Verification items for the finished model (mm, model axes). Face numbers are marked on the shaded views. A direction names the side the tool comes from. Give positions to 0.01 mm unless a question says otherwise; leave off trailing zeros. Loops run counter-clockwise (first coordinate to the right, second up) from the corner with the lowest first, then second, coordinate; pieces in that order, holes last. Notation, with made-up numbers: M 28,-37 L 36,-37 A23 cw 36,-10 Z; hole C -14.5,-8 d5. An arc over 180 degrees is marked long. Use CSV: the item, a comma, the result in double quotes.
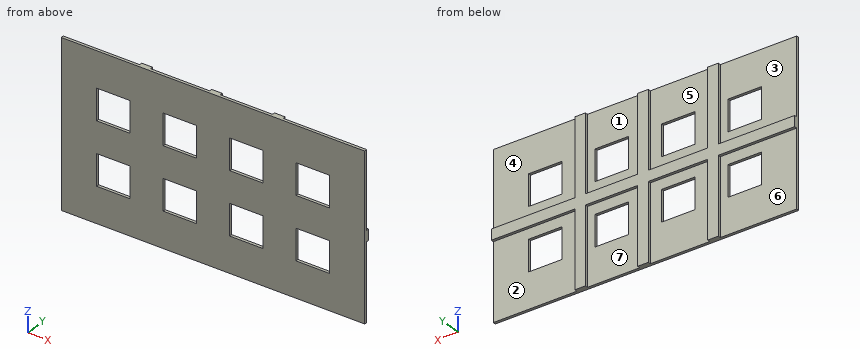
Autodesk Inventor part; units mm, degrees
ref_plane "YZ Plane" through (0, 0, 0) normal (1, 0, 0) x (0, 1, 0)
ref_plane "XZ Plane" through (0, 0, 0) normal (0, 1, 0) x (-1, 0, 0)
ref_plane "XY Plane" through (0, 0, 0) normal (0, 0, 1) x (1, 0, 0)
sketch "Sketch1" plane through (0, 0, 0) normal (0, 1, 0) x (-1, 0, 0)
  line L0 (0, 0) -> (-25.4, 0) construction
  line L1 (-25.4, 0) -> (-25.4, -25.4) construction
  line L2 (-25.4, -25.4) -> (0, -25.4) construction
  line L3 (0, -25.4) -> (0, 0) construction
  line L4 (-25.4, -25.4) -> (-49.2125, -25.4) construction
  line L5 (-49.2125, -25.4) -> (-49.2125, -47.625) construction
  line L6 (-49.2125, -47.625) -> (-25.4, -47.625) construction
  line L7 (-25.4, -47.625) -> (-25.4, -25.4) construction
  line L8 (-73.025, -25.4) -> (-96.8375, -25.4) construction
  line L9 (-96.8375, -25.4) -> (-96.8375, -47.625) construction
  line L10 (-96.8375, -47.625) -> (-73.025, -47.625) construction
  line L11 (-73.025, -47.625) -> (-73.025, -25.4) construction
  line L12 (-120.65, -25.4) -> (-144.4625, -25.4) construction
  line L13 (-144.4625, -25.4) -> (-144.4625, -47.625) construction
  line L14 (-144.4625, -47.625) -> (-120.65, -47.625) construction
  line L15 (-120.65, -47.625) -> (-120.65, -25.4) construction
  line L16 (-168.275, -25.4) -> (-192.0875, -25.4) construction
  line L17 (-192.0875, -25.4) -> (-192.0875, -47.625) construction
  line L18 (-192.0875, -47.625) -> (-168.275, -47.625) construction
  line L19 (-168.275, -47.625) -> (-168.275, -25.4) construction
  line L20 (-25.4, -69.85) -> (-49.2125, -69.85) construction
  line L21 (-49.2125, -69.85) -> (-49.2125, -92.075) construction
  line L22 (-49.2125, -92.075) -> (-25.4, -92.075) construction
  line L23 (-25.4, -92.075) -> (-25.4, -69.85) construction
  line L24 (-73.025, -69.85) -> (-96.8375, -69.85) construction
  line L25 (-96.8375, -69.85) -> (-96.8375, -92.075) construction
  line L26 (-96.8375, -92.075) -> (-73.025, -92.075) construction
  line L27 (-73.025, -92.075) -> (-73.025, -69.85) construction
  line L28 (-120.65, -69.85) -> (-144.4625, -69.85) construction
  line L29 (-144.4625, -69.85) -> (-144.4625, -92.075) construction
  line L30 (-144.4625, -92.075) -> (-120.65, -92.075) construction
  line L31 (-120.65, -92.075) -> (-120.65, -69.85) construction
  line L32 (-168.275, -69.85) -> (-192.0875, -69.85) construction
  line L33 (-192.0875, -69.85) -> (-192.0875, -92.075) construction
  line L34 (-192.0875, -92.075) -> (-168.275, -92.075) construction
  line L35 (-168.275, -92.075) -> (-168.275, -69.85) construction
  line L36 (-192.0875, -92.075) -> (-217.4875, -92.075) construction
  line L37 (-217.4875, -92.075) -> (-217.4875, -117.475) construction
  line L38 (-217.4875, -117.475) -> (-192.0875, -117.475) construction
  line L39 (-192.0875, -117.475) -> (-192.0875, -92.075) construction
  line L40 (0, 0) -> (-217.4875, 0)
  line L41 (-217.4875, 0) -> (-217.4875, -117.475)
  line L42 (-217.4875, -117.475) -> (0, -117.475)
  line L43 (0, -117.475) -> (0, 0)
  line L44 (-192.0875, -92.075) -> (-168.275, -92.075)
  line L45 (-168.275, -92.075) -> (-168.275, -69.85)
  line L46 (-168.275, -69.85) -> (-192.0875, -69.85)
  line L47 (-192.0875, -69.85) -> (-192.0875, -92.075)
  line L48 (-144.4625, -92.075) -> (-120.65, -92.075)
  line L49 (-120.65, -92.075) -> (-120.65, -69.85)
  line L50 (-120.65, -69.85) -> (-144.4625, -69.85)
  line L51 (-144.4625, -69.85) -> (-144.4625, -92.075)
  line L52 (-96.8375, -92.075) -> (-73.025, -92.075)
  line L53 (-73.025, -92.075) -> (-73.025, -69.85)
  line L54 (-73.025, -69.85) -> (-96.8375, -69.85)
  line L55 (-96.8375, -69.85) -> (-96.8375, -92.075)
  line L56 (-49.2125, -92.075) -> (-25.4, -92.075)
  line L57 (-25.4, -92.075) -> (-25.4, -69.85)
  line L58 (-25.4, -69.85) -> (-49.2125, -69.85)
  line L59 (-49.2125, -69.85) -> (-49.2125, -92.075)
  line L60 (-25.4, -47.625) -> (-49.2125, -47.625)
  line L61 (-49.2125, -47.625) -> (-49.2125, -25.4)
  line L62 (-49.2125, -25.4) -> (-25.4, -25.4)
  line L63 (-25.4, -25.4) -> (-25.4, -47.625)
  line L64 (-73.025, -47.625) -> (-96.8375, -47.625)
  line L65 (-96.8375, -47.625) -> (-96.8375, -25.4)
  line L66 (-96.8375, -25.4) -> (-73.025, -25.4)
  line L67 (-73.025, -25.4) -> (-73.025, -47.625)
  line L68 (-120.65, -47.625) -> (-144.4625, -47.625)
  line L69 (-144.4625, -47.625) -> (-144.4625, -25.4)
  line L70 (-144.4625, -25.4) -> (-120.65, -25.4)
  line L71 (-120.65, -25.4) -> (-120.65, -47.625)
  line L72 (-168.275, -47.625) -> (-192.0875, -47.625)
  line L73 (-192.0875, -47.625) -> (-192.0875, -25.4)
  line L74 (-192.0875, -25.4) -> (-168.275, -25.4)
  line L75 (-168.275, -25.4) -> (-168.275, -47.625)
  dimension "d1" = 25.4
  dimension "d2" = 23.8125
  dimension "d3" = 22.225
  dimension "d6" = 47.625
  dimension "d9" = 44.45
  dimension "d12" = 25.4
  dimension "d13" = 25.4
extrude "Extrusion1" add sketch "Sketch1" along normal blind 2
sketch "Sketch2" plane through (0, 2, 0) normal (0, 1, 0) x (1, 0, 0)
  line L0 (217.4875, 0) -> (217.4875, 117.475) construction
  line L1 (217.4875, 117.475) -> (0, 117.475) construction
  line L2 (0, 117.475) -> (0, 0) construction
  line L3 (0, 0) -> (217.4875, 0) construction
  line L4 (168.275, 47.625) -> (192.0875, 47.625) construction
  line L5 (192.0875, 47.625) -> (192.0875, 25.4) construction
  line L6 (192.0875, 25.4) -> (168.275, 25.4) construction
  line L7 (168.275, 25.4) -> (168.275, 47.625) construction
  line L8 (120.65, 47.625) -> (144.4625, 47.625) construction
  line L9 (144.4625, 47.625) -> (144.4625, 25.4) construction
  line L10 (144.4625, 25.4) -> (120.65, 25.4) construction
  line L11 (120.65, 25.4) -> (120.65, 47.625) construction
  line L12 (73.025, 47.625) -> (96.8375, 47.625) construction
  line L13 (96.8375, 47.625) -> (96.8375, 25.4) construction
  line L14 (96.8375, 25.4) -> (73.025, 25.4) construction
  line L15 (73.025, 25.4) -> (73.025, 47.625) construction
  line L16 (25.4, 47.625) -> (49.2125, 47.625) construction
  line L17 (49.2125, 47.625) -> (49.2125, 25.4) construction
  line L18 (49.2125, 25.4) -> (25.4, 25.4) construction
  line L19 (25.4, 25.4) -> (25.4, 47.625) construction
  line L20 (49.2125, 92.075) -> (49.2125, 69.85) construction
  line L21 (49.2125, 69.85) -> (25.4, 69.85) construction
  line L22 (25.4, 69.85) -> (25.4, 92.075) construction
  line L23 (25.4, 92.075) -> (49.2125, 92.075) construction
  line L24 (96.8375, 92.075) -> (96.8375, 69.85) construction
  line L25 (96.8375, 69.85) -> (73.025, 69.85) construction
  line L26 (73.025, 69.85) -> (73.025, 92.075) construction
  line L27 (73.025, 92.075) -> (96.8375, 92.075) construction
  line L28 (144.4625, 92.075) -> (144.4625, 69.85) construction
  line L29 (144.4625, 69.85) -> (120.65, 69.85) construction
  line L30 (120.65, 69.85) -> (120.65, 92.075) construction
  line L31 (120.65, 92.075) -> (144.4625, 92.075) construction
  line L32 (192.0875, 92.075) -> (192.0875, 69.85) construction
  line L33 (192.0875, 69.85) -> (168.275, 69.85) construction
  line L34 (168.275, 69.85) -> (168.275, 92.075) construction
  line L35 (168.275, 92.075) -> (192.0875, 92.075) construction
  line L36 (0, 54.9275) -> (217.4875, 54.9275) construction
  line L37 (217.4875, 54.9275) -> (217.4875, 62.5475) construction
  line L38 (217.4875, 62.5475) -> (0, 62.5475) construction
  line L39 (0, 62.5475) -> (0, 54.9275) construction
  line L40 (0, 54.9275) -> (217.4875, 62.5475) construction
  line L41 (217.4875, 54.9275) -> (0, 62.5475) construction
  line L42 (104.9338, 0) -> (112.5538, 0) construction
  line L43 (112.5538, 0) -> (112.5537, 117.475) construction
  line L44 (112.5537, 117.475) -> (104.9337, 117.475) construction
  line L45 (104.9337, 117.475) -> (104.9338, 0) construction
  line L46 (104.9338, 0) -> (112.5537, 117.475) construction
  line L47 (112.5538, 0) -> (104.9337, 117.475) construction
  line L48 (0, 62.5475) -> (217.4875, 62.5475)
  line L49 (217.4875, 62.5475) -> (217.4875, 54.9275)
  line L50 (217.4875, 54.9275) -> (0, 54.9275)
  line L51 (0, 54.9275) -> (0, 62.5475)
  line L52 (104.9337, 117.475) -> (112.5537, 117.475)
  line L53 (112.5537, 117.475) -> (112.5538, 0)
  line L54 (112.5538, 0) -> (104.9338, 0)
  line L55 (104.9338, 0) -> (104.9337, 117.475)
  line L56 (49.2125, 92.075) -> (73.025, 92.075) construction
  line L57 (73.025, 92.075) -> (73.025, 69.85) construction
  line L58 (73.025, 69.85) -> (49.2125, 69.85) construction
  line L59 (49.2125, 69.85) -> (49.2125, 92.075) construction
  line L60 (168.275, 92.075) -> (144.4625, 92.075) construction
  line L61 (144.4625, 92.075) -> (144.4625, 69.85) construction
  line L62 (144.4625, 69.85) -> (168.275, 69.85) construction
  line L63 (168.275, 69.85) -> (168.275, 92.075) construction
  line L64 (217.4875, 117.475) -> (0, 117.475)
  line L65 (54.7688, 0) -> (62.3888, 0)
  line L66 (62.3888, 0) -> (62.3888, 117.475)
  line L67 (62.3888, 117.475) -> (54.7688, 117.475)
  line L68 (54.7688, 117.475) -> (54.7688, 0)
  line L69 (54.7688, 0) -> (62.3888, 117.475) construction
  line L70 (62.3888, 0) -> (54.7688, 117.475) construction
  line L71 (150.0187, 0) -> (157.6388, 0)
  line L72 (157.6388, 0) -> (157.6387, 117.475)
  line L73 (157.6387, 117.475) -> (150.0187, 117.475)
  line L74 (150.0187, 117.475) -> (150.0187, 0)
  line L75 (150.0187, 0) -> (157.6387, 117.475) construction
  line L76 (157.6388, 0) -> (150.0187, 117.475) construction
  point P0 (108.7438, 58.7375)
  point P1 (108.7438, 58.7375)
  point P2 (58.5787, 58.7375)
  point P3 (153.8288, 58.7375)
  point P4 (54.7688, 54.9275)
  point P5 (62.3888, 54.9275)
  point P6 (104.9338, 54.9275)
  point P7 (112.5538, 54.9275)
  point P8 (150.0187, 54.9275)
  point P9 (157.6388, 54.9275)
  point P10 (157.6388, 62.5475)
  point P11 (150.0187, 62.5475)
  point P12 (112.5537, 62.5475)
  point P13 (104.9338, 62.5475)
  point P14 (62.3888, 62.5475)
  point P15 (54.7688, 62.5475)
  dimension "d16" = 7.62
  dimension "d17" = 7.62
  dimension "d18" = 7.62
  dimension "d19" = 7.62
extrude "Extrusion2" add sketch "Sketch2" along normal blind 2 contours L48 L68 L50 L51 | L68 L64 L66 L48 | L48 L66 L50 L68 | L48 L55 L50 L66 | L50 L66 L65 L68 | L55 L52 L53 L48 | L48 L53 L50 L55 | L48 L74 L50 L53 | L50 L53 L54 L55 | L74 L64 L72 L48 | L48 L72 L50 L74 | L48 L49 L50 L72 | L50 L72 L71 L74
properties part number "test_front_cover"
(1) Scan lines: L1, parallel to X at y = 2.5, z = -66.5; L2, parallel to Z at x = 132.5, y = 1.1 (3 decimals); L3, parallel to Z at x = 201, y = 3.05. Record each from-to range of solid material in increasing order. Write a range as from..to.
Calculated:
L1,"x = 54.77..62.39, 104.93..112.55, 150.02..157.64"
L2,"z = -117.475..-92.075, -69.85..-47.625, -25.4..0"
L3,"z = -62.55..-54.93"
(2) Section check D-D on z = -14. Record the cut outline in (x, y).
Calculated:
outline,"M 0,0 L 217.49,0 L 217.49,2 L 157.64,2 L 157.64,4 L 150.02,4 L 150.02,2 L 112.55,2 L 112.55,4 L 104.93,4 L 104.93,2 L 62.39,2 L 62.39,4 L 54.77,4 L 54.77,2 L 0,2 Z"
(3) Mould release check, pull along X, two halves, no side actions. Record for the marked faces 1 and 2: released by +X, released by -X, zero draft, split by the parting line, or undercut.
Calculated:
face 1,"undercut"
face 2,"zero draft"
(4) Section check A-A on x = 142. Count the separate pieces of the cut face and the enclosed holes in it, plus the area to 3 significant figures.
Calculated:
separate pieces,"3"
enclosed holes,"0"
area,"161 mm²"
(5) Section check C-C on x = 202. Record the cut outline in (y, z) (1 decimal), plus the area to 3 significant figures.
Calculated:
outline,"M 0,-117.5 L 2,-117.5 L 2,-62.5 L 4,-62.5 L 4,-54.9 L 2,-54.9 L 2,0 L 0,0 Z"
area,"250 mm²"
(6) Tool access check on the marked faces 3, 4, 5, 6 and 7. Record the directions out of +Z, -Z, +X, -X, +Y, -Y that give a thin tool (end or side, any length) a straight path to the whole face; none if there is none.
Calculated:
face 3,"+Z, -X, +Y"
face 4,"+Z, +X, +Y"
face 5,"+Z, +Y"
face 6,"-Z, -X, +Y"
face 7,"-Z, +Y"
(7) Depth check by flat-ended pin: pin 1 Ø0.6 at (y, z) = (3.5, -96.5) entering from +X; pin 2 Ø0.6 at (x, y) = (36, 3) entering from -Z; pin 3 Ø1.6 at (y, z) = (3, -30.5) entering from -X. Enter the tip coordinate at first touch or a pass-through.
Calculated:
pin 1,"stops at x = 157.64"
pin 2,"stops at z = -62.55"
pin 3,"stops at x = 54.77"
